Could you check a few things on this model? Use its own coordinates, in mm. Face numbers are marked on the shaded views. Round coordinates to 2 decimals unless told otherwise and drop trailing zeros. Order: outer loops, then holes, each group sorted by start corner. A loop starts at its lowest first (then second) coordinate and runs counter-clockwise, first axis right, second up. Notation, with made-up numbers: (80.5, 81) -> (126.5, 81) arc R24 ccw to (126.5, 92) -> close; hole circle Ø1 at (85.5, 25). An arc over 180 degrees is marked (long way). One line per question, with ' | ' between items.
```python
from build123d import *

# Parameters (mm, degrees)
SZKIC1_W                    = 14
SZKIC1_H                    = 3
SZKIC4_R                    = 10.5
DODANIE_WYCI_GNI_CIE1_DEPTH = 7


with BuildPart() as part:
    # Szkic1 → Obrót1 (revolve)
    with BuildSketch(Plane(origin=(0, 0, 0), x_dir=(1, 0, 0), z_dir=(0, 1, 0)), mode=Mode.PRIVATE) as obr_t1_sk:
        with Locations((7, -1.5)):
            Rectangle(SZKIC1_W, SZKIC1_H)
    revolve(obr_t1_sk.sketch.rotate(Axis((0, 0, 3), (0, 0, -1)), 180), axis=Axis((0, 0, 3), (0, 0, -1)))

    # Szkic2 → Wycięcie-obrót1 (revolve, cut)
    with BuildSketch(Plane(origin=(0, 0, 0), x_dir=(1, 0, 0), z_dir=(0, 1, 0)), mode=Mode.PRIVATE) as wyci_cie_obr_t1_sk:
        Polygon((13, -3), (14, -3), (14, -2), align=None)
    revolve(wyci_cie_obr_t1_sk.sketch.rotate(Axis((0, 0, 3), (0, 0, -1)), 180), axis=Axis((0, 0, 3), (0, 0, -1)), mode=Mode.SUBTRACT)

    # Szkic3 → Wycięcie-obrót2 (revolve, cut)
    with BuildSketch(Plane(origin=(0, 0, 0), x_dir=(1, 0, 0), z_dir=(0, 1, 0)), mode=Mode.PRIVATE) as wyci_cie_obr_t2_sk:
        Polygon((0, 0), (2.15, 0), (2.15, -0.7), (4.45, -3), (0, -3), align=None)
    revolve(wyci_cie_obr_t2_sk.sketch.rotate(Axis((0, 0, 3), (0, 0, -1)), 180), axis=Axis((0, 0, 3), (0, 0, -1)), mode=Mode.SUBTRACT)


with BuildPart() as body_2:
    # Szkic4 → Dodanie-wyciągnięcie1 (new body)
    with BuildSketch(Plane(origin=(0, 0, 0), x_dir=(0, 0, -1), z_dir=(1, 0, 0))):
        Circle(SZKIC4_R)
    extrude(amount=DODANIE_WYCI_GNI_CIE1_DEPTH)

    # Usuń ścianę1: 1 face struck out; the rest of the skin is kept as a surface, the solid goes
    usu_cian_1_1_drop = [body_2.part.faces().sort_by_distance(Vector(p))[0] for p in ((7, 0, 0),)]
    usu_cian_1_1 = Shell(body_2.part.faces() - usu_cian_1_1_drop)


solid = part.part
```
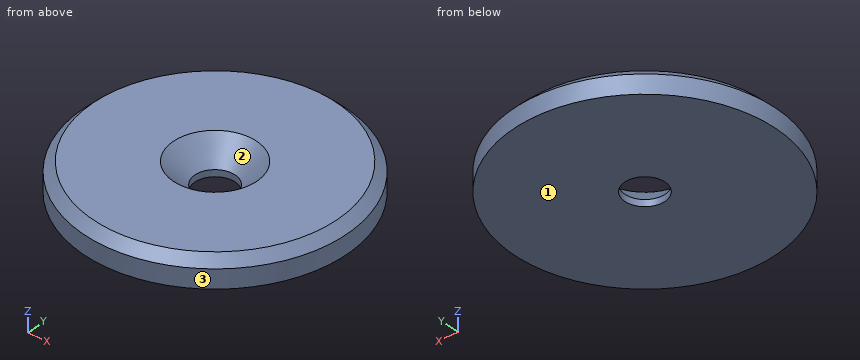
1. I'm going to push a flat-ended pin straight in: pin 1 (1 mm diameter, centred on y = 6, z = 1, fed in from -X). Where does the tip first touch, or does it pass through?
From the geometry:
pin 1: stops at x = -12.87
2. I need wall thicknesses on probe 1 along Y at (x, z) = (0, 0.5); probe 2 along X at (y, z) = (-3, 2); probe 3 along Y at (x, z) = (-1.5, 2.7). Which ranges of each line are inside material? Lowest first, please.
From the geometry:
probe 1: y = -14 to -2.15, 2.15 to 14 | probe 2: x = -13.67 to -1.7, 1.7 to 13.67 | probe 3: y = -13.22 to -3.87, 3.87 to 13.22
3. I want a section at A-A on x = 0. List the corners of the cut face in (y, z) for me, and give its area (3 significant figures).
From the geometry:
outline: (-14, 0) -> (-2.15, 0) -> (-2.15, 0.7) -> (-4.45, 3) -> (-13, 3) -> (-14, 2) -> close; (2.15, 0) -> (14, 0) -> (14, 2) -> (13, 3) -> (4.45, 3) -> (2.15, 0.7) -> close | area: 64.8 mm²
4. I want a section at C-C on z = 0.35. List the corners of the cut face in (x, y) for me, and give its area (3 significant figures).
From the geometry:
outline: circle Ø28 at (0, 0); hole circle Ø4.3 at (0, 0) | area: 601 mm²
5. I want a section at D-D on z = 2.45. List the corners of the cut face in (x, y) for me.
From the geometry:
outline: circle Ø27.1 at (0, 0); hole circle Ø7.8 at (0, 0)
6. If we mould it in two halves opening along Y, with no side actions, what happens to the marked faces 1, 2 and 3? For each: pulls with the +Y half, pulls with the -Y half, needs draft (parallel to the pull), parting line crosses it, or undercut.
From the geometry:
face 1: needs draft | face 2: undercut | face 3: parting line crosses it
